Check sheet for the modelled part. Datum: model origin and axes. Units: mm. A direction names the side the tool comes from. Give positions to 0.01 mm unless a question says otherwise; leave off trailing zeros. Order: outer loops, then holes, each group sorted by start corner. A loop starts at its lowest first (then second) coordinate and runs counter-clockwise, first axis right, second up. Notation, with made-up numbers: (69.25, 30.5) -> (113.25, 30.5) arc R22 ccw to (113.25, 41.5) -> close; hole circle Ø5 at (-2, 50). An arc over 180 degrees is marked (long way). One line per question, with ' | ' between items.
Autodesk Inventor part; units mm, degrees
ref_plane "Work Plane4" through (0, 0, 30.8) normal (0, 0, 1) x (1, 0, 0)
ref_plane "YZ Plane" through (0, 0, 0) normal (1, 0, 0) x (0, 1, 0)
ref_plane "XZ Plane" through (0, 0, 0) normal (0, 1, 0) x (-1, 0, 0)
sketch "Sketch15" plane through (0, 0, 0) normal (0, 1, 0) x (-1, 0, 0)
  line L0 (0, 0) -> (-13, 0)
  line L1 (-13, 0) -> (-13, 160)
  line L2 (-13, 160) -> (0, 160)
  line L3 (0, 160) -> (0, 0)
  line L4 (-13, 0) -> (-13, -1.5)
  line L5 (-13, -1.5) -> (0, -1.5)
  line L6 (0, -1.5) -> (0, 0)
  dimension "d75" = 13
  dimension "d76" = 160
  dimension "d127" = 1.5
extrude "Extrusion15" add sketch "Sketch15" along normal blind 2
sketch "Sketch16" plane through (0, 2, 0) normal (0, 1, 0) x (1, 0, 0)
  line L0 (0, 0) -> (0, -160)
  line L1 (13, -160) -> (13, 1.5)
  line L2 (0, -160) -> (13, -160)
  line L3 (13, -160) -> (13, -155.5)
  line L4 (13, -155.5) -> (0, -155.5)
  line L5 (0, -155.5) -> (0, -160)
  circle A0 centre (6.5, -157.75) radius 1.4
  circle A1 centre (6.5, -129.95) radius 1.4
  line L6 (13, -127.7) -> (13, -132.2)
  line L7 (13, -132.2) -> (0, -132.2)
  line L8 (0, -127.7) -> (13, -127.7)
  line L9 (0, -127.7) -> (0, -132.2)
  point P0 (20, 0)
  point P1 (13, -160)
  point P2 (0, -155.5)
  point P3 (13, 1.5)
extrude "Extrusion16" add sketch "Sketch16" along normal blind 17.25 contours L8 L1 L7 L0 | L4 L1 L2 L0 | A0 | A1
sketch "Sketch20" plane through (0, 2, 0) normal (0, 1, 0) x (1, 0, 0)
  line L0 (0, -127.7) -> (13, -127.7)
  line L1 (0, -127.7) -> (0, -123.2)
  line L2 (0, 0) -> (0, -127.7)
  line L3 (0, -123.2) -> (13, -123.2)
  line L4 (13, -127.7) -> (13, 1.5)
  line L5 (13, -127.7) -> (13, -123.2)
  line L6 (13, -132.2) -> (13, -127.7)
  line L7 (13, -127.7) -> (0, -127.7)
  circle A0 centre (6.5, -125.45) radius 1.4
  circle A1 centre (6.5, -97.65) radius 1.4
  line L8 (10, -95.4) -> (13, -95.4)
  line L9 (13, -95.4) -> (13, -99.9)
  line L10 (13, -99.9) -> (0, -99.9)
  line L11 (0, -95.4) -> (10, -95.4)
  line L12 (0, -95.4) -> (0, -99.9)
  line L13 (6.5, -123.2) -> (6.5, -125.45)
  point P0 (20, 0)
  point P1 (13, 1.5)
  dimension "d95" = 4.5
  dimension "d96" = 2.8
extrude "Extrusion20" add sketch "Sketch20" along normal blind 22.25 contours A0 | L1 L3 L4 L0 | L2 L11 L8 L4 L10 | A1
sketch "Sketch21" plane through (0, 2, 0) normal (0, 1, 0) x (1, 0, 0)
  line L0 (13, -95.4) -> (0, -95.4)
  line L1 (0, -95.4) -> (0, -90.9)
  line L2 (0, 0) -> (0, -160)
  line L3 (13, -160) -> (13, 1.5)
  line L4 (0, -95.4) -> (13, -95.4)
  circle A0 centre (6.5, -93.15) radius 1.4
  circle A1 centre (6.5, -65.35) radius 1.4
  line L5 (10, -63.1) -> (13, -63.1)
  line L6 (13, -63.1) -> (13, -67.6)
  line L7 (13, -67.6) -> (0, -67.6)
  line L8 (0, -67.6) -> (0, -63.1)
  line L9 (0, -63.1) -> (10, -63.1)
  line L10 (13, -95.4) -> (13, -90.9)
  line L11 (0, -90.9) -> (13, -90.9)
  point P0 (20, -90.9)
  point P1 (20, 0)
  point P2 (13, 1.5)
  dimension "d102" = 4.5
extrude "Extrusion21" add sketch "Sketch21" along normal blind 27.25 contours L0 L1 L11 L3 | L7 L2 L9 L5 L3 | A0 | A1
sketch "Sketch22" plane through (0, 2, 0) normal (0, 1, 0) x (1, 0, 0)
  line L0 (0, -63.1) -> (13, -63.1)
  line L1 (0, -63.1) -> (0, -58.6)
  line L2 (0, 0) -> (0, -160)
  line L3 (0, -58.6) -> (13, -58.6)
  line L4 (13, -160) -> (13, 1.5)
  line L5 (13, -58.6) -> (13, -63.1)
  line L6 (13, -63.1) -> (0, -63.1)
  circle A0 centre (6.5, -60.85) radius 1.4
  circle A1 centre (6.5, -33.05) radius 1.4
  line L7 (10, -30.8) -> (13, -30.8)
  line L8 (13, -30.8) -> (13, -35.3)
  line L9 (13, -35.3) -> (0, -35.3)
  line L10 (0, -30.8) -> (0, -35.3)
  line L11 (0, -30.8) -> (10, -30.8)
  line L12 (6.5, -58.6) -> (6.5, -60.85)
  point P0 (20, 0)
  point P1 (13, 1.5)
  dimension "d110" = 4.5
  dimension "d111" = 2.8
extrude "Extrusion22" add sketch "Sketch22" along normal blind 32.25 contours A0 | L1 L3 L4 L0 | L2 L11 L7 L4 L9 | A1
sketch "Sketch23" plane through (0, 2, 0) normal (0, 1, 0) x (1, 0, 0)
  line L0 (0, -30.8) -> (13, -30.8)
  line L1 (0, -30.8) -> (0, -26.3)
  line L2 (0, 0) -> (0, -160)
  line L3 (0, -26.3) -> (13, -26.3)
  line L4 (13, -160) -> (13, 1.5)
  line L5 (13, -26.3) -> (13, -30.8)
  line L6 (13, -30.8) -> (0, -30.8)
  circle A0 centre (6.5, -28.55) radius 1.4
  circle A1 centre (6.5, -0.75) radius 1.4
  line L7 (20, 0) -> (0, 0)
  line L8 (3, 1.5) -> (13, 1.5)
  line L9 (13, 1.5) -> (13, -3)
  line L10 (13, -3) -> (0, -3)
  line L11 (0, -3) -> (0, 1.5)
  line L12 (0, 1.5) -> (3, 1.5)
  line L13 (6.5, -26.3) -> (6.5, -28.55)
  dimension "d118" = 4.5
  dimension "d119" = 2.8
  dimension "d124" = 4.5
extrude "Extrusion23" add sketch "Sketch23" along normal blind 37.25 contours A0 | L1 L3 L4 L0 | L2 L7 A1 L4 L10 | L11 L12 L8 L4 L7 A1 | L7 A1 | A1 L7
sketch "Sketch27" plane through (0, 2, 0) normal (0, 1, 0) x (1, 0, 0)
  line L0 (0, -123.2) -> (13, -123.2)
  line L1 (0, -99.9) -> (13, -99.9)
  line L2 (0, -123.2) -> (13, -123.2)
  line L3 (13, -123.2) -> (13, -99.9)
  line L4 (13, -99.9) -> (0, -99.9)
  line L5 (0, -99.9) -> (0, -123.2)
  point P0 (0, 0)
extrude "Extrusion27" add sketch "Sketch27" along normal blind 5
sketch "Sketch28" plane through (0, 2, 0) normal (0, 1, 0) x (1, 0, 0)
  line L0 (13, -90.9) -> (13, -67.6)
  line L1 (0, -67.6) -> (0, -90.9)
  line L2 (13, -90.9) -> (0, -90.9)
  line L3 (0, -90.9) -> (0, -67.6)
  line L4 (0, -67.6) -> (13, -67.6)
  line L5 (13, -67.6) -> (13, -90.9)
  point P0 (0, 0)
extrude "Extrusion28" add sketch "Sketch28" along normal blind 10
sketch "Sketch29" plane through (0, 2, 0) normal (0, 1, 0) x (1, 0, 0)
  line L0 (13, -58.6) -> (0, -58.6)
  line L1 (0, -58.6) -> (13, -58.6)
  line L2 (13, -58.6) -> (13, -35.3)
  line L3 (13, -35.3) -> (0, -35.3)
  line L4 (0, -35.3) -> (0, -58.6)
  point P0 (0, 0)
extrude "Extrusion29" add sketch "Sketch29" along normal blind 15
sketch "Sketch30" plane through (0, 2, 0) normal (0, 1, 0) x (1, 0, 0)
  line L0 (0, -26.3) -> (13, -26.3)
  line L1 (0, -3) -> (13, -3)
  line L2 (0, -26.3) -> (13, -26.3)
  line L3 (13, -26.3) -> (13, -3)
  line L4 (13, -3) -> (0, -3)
  line L5 (0, -3) -> (0, -26.3)
  point P0 (0, 0)
extrude "Extrusion30" add sketch "Sketch30" along normal blind 20
ref_plane "Work Plane1" through (0, 0, -1.5) normal (0, 0, 1) x (1, 0, 0)
ref_plane "Work Plane4" through (0, 0, 30.8) normal (0, 0, 1) x (1, 0, 0)
ref_plane "Work Plane3" through (0, 0, 95.4) normal (0, 0, 1) x (1, 0, 0)
sketch "Sketch35" plane through (0, 19.25, 0) normal (0, 1, 0) x (1, 0, 0)
  line L0 (0, -160) -> (13, -160)
  line L1 (6.5, -160) -> (6.5, -157.75)
  line L2 (6.5, -157.75) -> (6.5, -129.95)
  point P0 (0, 0)
  dimension "d168" = 2.25
  dimension "d169" = 27.8
hole "Hole1" at (6.5, 19.25, 129.95) at (6.5, 19.25, 157.75) direction (0, -1, 0) diameter 2.8 depth 3
sketch "Sketch36" plane through (0, 24.25, 0) normal (0, 1, 0) x (1, 0, 0)
  line L0 (0, -127.7) -> (13, -127.7)
  line L1 (6.5, -127.7) -> (6.5, -125.45)
  line L2 (6.5, -125.45) -> (6.5, -97.65)
  point P0 (0, 0)
hole "Hole2" at (6.5, 24.25, 125.45) at (6.5, 24.25, 97.65) direction (0, -1, 0) diameter 2.8 depth 3
sketch "Sketch37" plane through (0, 29.25, 0) normal (0, 1, 0) x (1, 0, 0)
  line L0 (0, -95.4) -> (13, -95.4)
  line L1 (6.5, -95.4) -> (6.5, -93.15)
  line L2 (6.5, -93.15) -> (6.5, -65.35)
  point P0 (0, 0)
hole "Hole3" at (6.5, 29.25, 93.15) at (6.5, 29.25, 65.35) direction (0, -1, 0) diameter 2.8 depth 3
sketch "Sketch38" plane through (0, 34.25, 0) normal (0, 1, 0) x (1, 0, 0)
  line L0 (0, -63.1) -> (13, -63.1)
  line L1 (6.5, -63.1) -> (6.5, -60.85)
  line L2 (6.5, -60.85) -> (6.5, -33.05)
  point P0 (0, 0)
  dimension "d195" = 2.25
  dimension "d196" = 27.8
hole "Hole4" at (6.5, 34.25, 60.85) at (6.5, 34.25, 33.05) direction (0, -1, 0) diameter 2.8 depth 3
sketch "Sketch39" plane through (0, 39.25, 0) normal (0, 1, 0) x (1, 0, 0)
  line L0 (13, -30.8) -> (0, -30.8)
  line L1 (6.5, -30.8) -> (6.5, -28.55)
  line L2 (6.5, -28.55) -> (6.5, -0.75)
  point P0 (0, 0)
  dimension "d204" = 2.25
  dimension "d205" = 27.8
hole "Hole5" at (6.5, 39.25, 28.55) at (6.5, 39.25, 0.75) direction (0, -1, 0) diameter 2.8 depth 3
thread "Thread1"
thread "Thread2"
thread "Thread3"
thread "Thread4"
thread "Thread5"
thread "Thread6"
thread "Thread7"
thread "Thread8"
thread "Thread9"
thread "Thread10"
ref_plane "Work Plane2" through (0, 0, 160) normal (0, 0, 1) x (1, 0, 0)
properties part number "Forearm_1" material "ABS Plastic"
Q1. Access from +Z, -Z, +X, -X, +Y, -Y to the whole of each face (thin tool, end or side, straight path). Record for faces 4 (the face through (6, 26.25, 93)), 5 (the face through (7, 0, 80)), 6 (the face through (5, 39.25, 29)), 7 (the face through (6, 19.25, 156)), 8 (the face through (6, 16, 123.2)).
Result sheet:
face 4: +Y | face 5: +Z, -Z, +X, -X, -Y | face 6: +Z, -Z, +X, -X, +Y | face 7: +Z, +X, -X, +Y | face 8: +X, -X, +Y
Q2. Section check A-A (z = 33.05). Enter the section's corners in (x, y), and give its area (3 significant figures).
Result sheet:
outline: (0, 0) -> (13, 0) -> (13, 34.25) -> (7.9, 34.25) -> (7.9, 31.25) -> (5.1, 31.25) -> (5.1, 34.25) -> (0, 34.25) -> close | area: 437 mm2
Q3. Depth check by flat-ended pin: pin 1 Ø6.5 at (x, z) = (3.5, 79.5) entering from +Y; pin 2 Ø5 at (x, z) = (6.5, 62) entering from +Y; pin 3 Ø6 at (x, z) = (2.5, 95) entering from +Y; pin 4 Ø6 at (y, z) = (29.5, 71.5) entering from -X. Enter the tip coordinate at first touch or a pass-through.
Result sheet:
pin 1: stops at y = 12 | pin 2: stops at y = 34.25 | pin 3: stops at y = 29.25 | pin 4: passes through
Q4. Section check D-D (z = 73.5). Enter the section's corners in (x, y), and give its area (3 significant figures).
Result sheet:
outline: (0, 0) -> (13, 0) -> (13, 12) -> (0, 12) -> close | area: 156 mm2
Q5. Mould release check, pull along Z, two halves, no side actions. Record for faces 1 (the face through (0, 11, 60)), 2 (the face through (6.44, 17.73, 156.35)), 3 (the face through (6, 22, 127.7)): pulls with the +Z half, pulls with the -Z half, needs draft (parallel to the pull), parting line crosses it, or undercut.
Result sheet:
face 1: needs draft | face 2: undercut | face 3: pulls with the +Z half
Q6. Thickness scan on line 1 (Z direction, x = 6.5, y = 37.9); line 2 (Z direction, x = 6.5, y = 28.65); line 3 (Z direction, x = 2.75, y = 14.5). Record the ranges inside material, lowest first.
Result sheet:
line 1: z = -1.5 to -0.65, 2.15 to 3, 26.3 to 27.15, 29.95 to 30.8 | line 2: z = -1.5 to 3, 26.3 to 35.3, 58.6 to 63.95, 66.75 to 67.6, 90.9 to 91.75, 94.55 to 95.4 | line 3: z = -1.5 to 67.6, 90.9 to 99.9, 123.2 to 132.2, 155.5 to 160
Q7. Section check C-C (z = 97.65). Enter the section's corners in (x, y).
Result sheet:
outline: (0, 0) -> (13, 0) -> (13, 24.25) -> (7.9, 24.25) -> (7.9, 21.25) -> (5.1, 21.25) -> (5.1, 24.25) -> (0, 24.25) -> close
